The model under review builds one solid part; all positions refer to its coordinate system, in mm. A direction names the side the tool comes from. Round coordinates to 2 decimals unless told otherwise and drop trailing zeros. Write each loop counter-clockwise with the first axis right and the second up, starting at its lowest first coordinate (ties: lowest second). Pieces come first, ordered by that corner, then holes. Notation, with made-up numbers: (63.5, 38.5) - (106.5, 38.5) arc R25 cw to (106.5, 67.5) - close; hole circle Ø8 at (29, -11). An arc over 180 degrees is marked (long way). Return JSON: item names as keys, results as strings.
Autodesk Inventor part; units mm, degrees
ref_plane "YZ Plane" through (0, 0, 0) normal (1, 0, 0) x (0, 1, 0)
ref_plane "XZ Plane" through (0, 0, 0) normal (0, 1, 0) x (-1, 0, 0)
ref_plane "XY Plane" through (0, 0, 0) normal (0, 0, 1) x (1, 0, 0)
sketch "Sketch1" plane through (0, 0, 0) normal (0, 0, 1) x (1, 0, 0)
  line L0 (0, -120) -> (0, 155.2673)
  line L1 (-130, 0) -> (-130, 5)
  line L2 (-10, 5) -> (0, 5)
  line L3 (0, -74) -> (-9.8, -74)
  line L4 (-130, 5) -> (-120, 5)
  line L5 (-120.2, -74) -> (-129.8, -74)
  line L6 (-129.8, -69) -> (-129.8, -74)
  line L7 (0, 5) -> (-170.1, 5)
  line L8 (-170.1, 5) -> (-170.1, -74)
  line L9 (-170.1, -74) -> (0, -74)
  line L10 (0, -74) -> (0, 5)
  line L11 (-156.6357, -1) -> (-156.6357, 5)
  line L12 (-170.1, -1) -> (-170.1, 5)
  point P0 (0, 0)
  dimension "d27" = 0
extrude "Extrusion1" add sketch "Sketch1" along normal blind 6
sketch "Sketch2" plane through (0, 0, 6) normal (0, 0, 1) x (1, 0, 0)
  line L0 (-10, 0) -> (-10, 5)
  line L1 (0, 5) -> (-170.1, 5)
  line L2 (-20, 0) -> (-10, 0)
  line L3 (-20, 5) -> (-20, 0)
  line L4 (-9.9, 5) -> (-9.9, 0)
  line L5 (-20.1, 0) -> (-20.1, 5)
  line L6 (-10, 0) -> (-9.9, 0)
  line L7 (-20, 0) -> (-20.1, 0)
  point P0 (-130, 5)
extrude "Extrusion2" cut sketch "Sketch2" against normal blind 6
sketch "Sketch3" plane through (-20.1, 0, 6) normal (0, 1, 0) x (1, 0, 0)
  circle A0 centre (5.1, 3) radius 1.5
  point P0 (20.1, 6)
hole "Hole1" at (-15, 0, 3) direction (0, -1, 0) diameter 2.8 depth 20
pattern_linear "Rectangular Pattern2" count 9 spacing 20 along (-1, 0, 0) of "Extrusion2", "Hole1"
ref_plane "Work Plane1" through (-170.1, -34.5, 0) normal (0, -1, 0) x (1, 0, 0)
mirror "Mirror1" about plane through (-170.1, -34.5, 0) normal (0, -1, 0) of "Extrusion2", "Hole1", "Rectangular Pattern2"
sketch "Skizze4" plane through (0, 0, 6) normal (0, 0, 1) x (1, 0, 0)
  line L0 (-3.4696, 5) -> (-3.4696, -74)
  line L1 (15.4076, -81.7963) -> (-3.9696, -81.7963)
  line L2 (-3.9696, -81.7963) -> (-3.9696, 13.3495)
  line L3 (-3.9696, 13.3495) -> (15.4076, 13.3495)
  line L4 (15.4076, 13.3495) -> (15.4076, -81.7963)
  point P0 (0, 0)
  dimension "d23" = 0.5
extrude "Extrusion3" cut sketch "Skizze4" against normal blind 10
sketch "Skizze5" plane through (0, 0, 6) normal (0, 0, 1) x (1, 0, 0)
  ellipse E0 centre (-101.986, -20.3375) end of major axis (-101.986, -27.7035) minor radius 7.2541
  ellipse E1 centre (-140.4361, -58.0565) end of major axis (-140.4361, -65.4225) minor radius 7.2541
  line L0 (-150.4361, -68.0565) -> (-91.986, -68.0565)
  line L1 (-86.986, -21.3155) -> (-86.986, -5)
  line L2 (-86.986, -5) -> (-150.4361, -5)
  line L3 (-150.4361, -5) -> (-150.4361, -68.0565)
  line L4 (-133.727, -68.0565) -> (-86.986, -21.3155)
  line L5 (-133.727, -68.0565) -> (-67.6252, -68.0565) construction
  line L6 (-86.986, -5) -> (-150.4361, -5)
  line L7 (-150.4361, -5) -> (-150.4361, -10)
  line L8 (-150.4361, -10) -> (-86.986, -10)
  line L9 (-86.986, -10) -> (-86.986, -5)
  point P0 (0, 0)
  dimension "d28" = 15
  dimension "d29" = 10
  dimension "d30" = 10
  dimension "d33" = 45
  dimension "d34" = 5
extrude "Extrusion4" cut sketch "Skizze5" against normal blind 10 contours E0 | E1 | L3 L8 L1 L4 L0
fillet "Rundung1" radius 3 4 edges at (-86.986, -10, 3) (-86.986, -21.3155, 3) (-150.4361, -68.0565, 3) (-150.4361, -10, 3)
properties part number "00_Baseplate_Simmo_side2"
(1) Clearance check with flat-ended pins moving along their axes: pin 1 Ø3 at (x, z) = (-75, 3) entering from -Y; pin 2 Ø2 at (x, z) = (-154.5, 3) entering from +Y; pin 3 Ø0.8 at (x, z) = (-35.5, 2.5) entering from -Y. State where each tip first meets the part, or that it passes through.
Filled in:
{"pin 1": "stops at y = -69", "pin 2": "stops at y = 0", "pin 3": "stops at y = -49"}
(2) For faces 3 (the flat face through (-100.1, 2, 3)), 4 (the flat face through (-86.986, -17, 3)), 5 (the flat face through (-155, -49, 3)), list the 3-axis set-ups (+Z, -Z, +X, -X, +Y, -Y) from which the entire face can be reached by the end or side of a thin tool; tool diameter is ignored.
Filled in:
{"face 3": "+Z, -Z, +Y", "face 4": "+Z, -Z", "face 5": "-Y"}
(3) Add section C-C (y = -28). Write out the cut boundary in (x, z).
Filled in:
{"outline": "(-170.1, 0) - (-150.44, 0) - (-150.44, 6) - (-170.1, 6) - close; (-93.67, 0) - (-3.97, 0) - (-3.97, 6) - (-93.67, 6) - close"}
(4) Add section B-B (y = -1.5). Give the number of separate pieces and of enclosed holes in the cut face, plus the area to 3 significant figures.
Filled in:
{"separate pieces": "1", "enclosed holes": "8", "area": "948 mm2"}
(5) Mouldability with a two-part tool opening along X and no side actions: class faces 1 (the cylindrical face through (-56.39, -10.14, 2.82)), 2 (the flat face through (-7, -74, 3)) as released by +X, released by -X, zero draft, split by the parting line, or undercut.
Filled in:
{"face 1": "undercut", "face 2": "zero draft"}
(6) Add section A-A (y = -42). Write out the cut boundary in (x, z), plus the area to 3 significant figures.
Filled in:
{"outline": "(-170.1, 0) - (-150.44, 0) - (-150.44, 6) - (-170.1, 6) - close; (-107.67, 0) - (-3.97, 0) - (-3.97, 6) - (-107.67, 6) - close", "area": "740 mm2"}
(7) Wall thickness on line 1 (Z direction, x = -35, y = -60.5); line 2 (Y direction, x = -59.5, z = 4.95); line 3 (X direction, y = -63, z = 0.55): over which ranges is each line inside the solid? List them lowest first.
Filled in:
{"line 1": "z = 0 to 1.6, 4.4 to 6", "line 2": "y = -69 to 0", "line 3": "x = -170.1 to -150.44, -128.67 to -3.97"}
